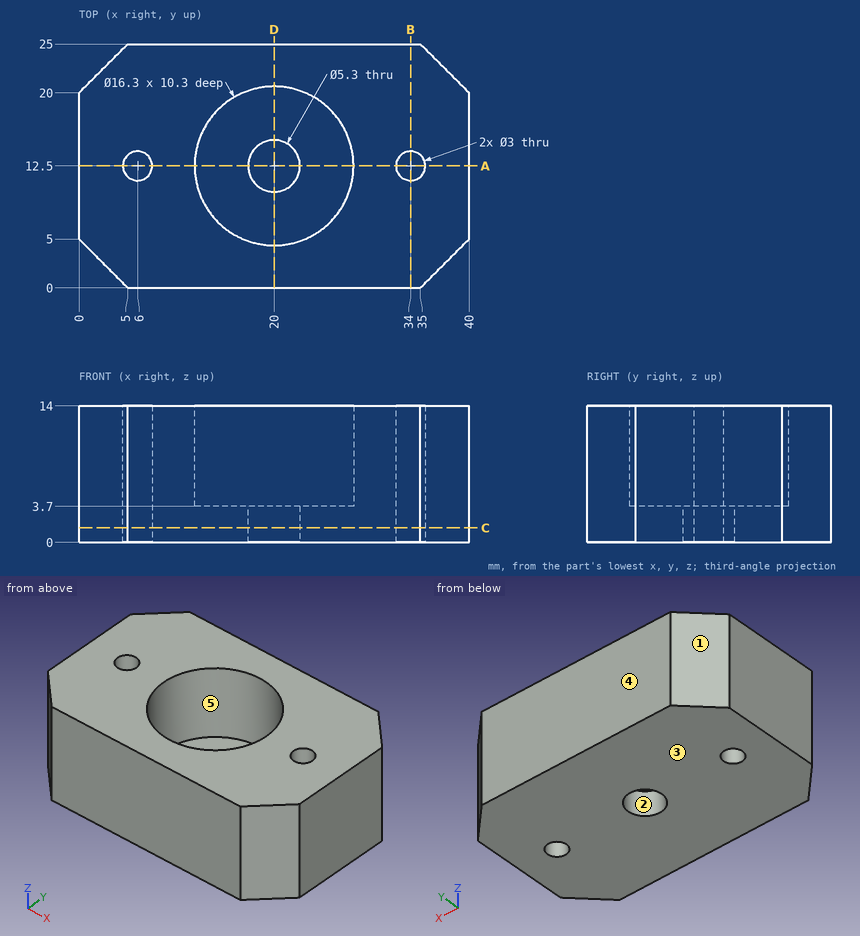
Check sheet for the drawn part. Datum: minimum x, y, z corner. Units: mm. A direction names the side the tool comes from. Coordinates: 2 decimals unless noted, no trailing zeros. Order: outer loops, then holes, each group sorted by start corner. A loop starts at its lowest first (then second) coordinate and runs counter-clockwise, first axis right, second up. Notation, with made-up numbers: M 27,80 L 65,80 A5 ccw 65,87 Z; hole C -34,82.25 d1. An arc over 180 degrees is marked long. One line per question, with ' | ' between items. Start each with the question number.
Item 1: Sectioned sample at B-B on x = 34. Record the cut outline in (y, z).
Item 2: Sectioned sample at C-C on z = 1.5. Record the cut outline in (x, y), and give its area (3 significant figures).
Item 3: Sectioned sample at A-A on y = 12.5. Record the cut outline in (x, z).
Item 4: Sectioned sample at D-D on x = 20. Record the cut outline in (y, z).
Item 5: Access from +Z, -Z, +X, -X, +Y, -Y to the whole of each face (thin tool, end or side, straight path). Record for the marked faces 4 and 5.
Item 6: Gauge pin test, flat ends, axial feed: P1, Ø2.5, axis at x = 6, y = 12.5, coming from the -Z side (3 decimals); P2, Ø7, axis at x = 20, y = 12.5, coming from the +Z side. Record the tip position at first contact, or that the pin passes through.
Item 7: Material ranges on line 1 (Y direction, x = 20, z = 10.25); line 2 (Y direction, x = 6, z = 10.25); line 3 (Z direction, x = 25.5, y = 13.5), recorded low to high.
Item 8: Mould release check, pull along Y, two halves, no side actions. Record for the marked faces 1, 2 and 3: pulls with the +Y half, pulls with the -Y half, needs draft (parallel to the pull), parting line crosses it, or undercut.
Answer below:
1) outline: M 0,0 L 11,0 L 11,14 L 0,14 Z; M 14,0 L 25,0 L 25,14 L 14,14 Z
2) outline: M 0,5 L 5,0 L 35,0 L 40,5 L 40,20 L 35,25 L 5,25 L 0,20 Z; hole C 6,12.5 d3; hole C 20,12.5 d5.3; hole C 34,12.5 d3 | area: 914 mm^2
3) outline: M 0,0 L 4.5,0 L 4.5,14 L 0,14 Z; M 7.5,0 L 17.35,0 L 17.35,3.7 L 11.85,3.7 L 11.85,14 L 7.5,14 Z; M 22.65,0 L 32.5,0 L 32.5,14 L 28.15,14 L 28.15,3.7 L 22.65,3.7 Z; M 35.5,0 L 40,0 L 40,14 L 35.5,14 Z
4) outline: M 0,0 L 9.85,0 L 9.85,3.7 L 4.35,3.7 L 4.35,14 L 0,14 Z; M 15.15,0 L 25,0 L 25,14 L 20.65,14 L 20.65,3.7 L 15.15,3.7 Z
5) face 4: +Z, -Z, +X, -X, +Y | face 5: +Z
6) P1: passes through | P2: stops at z = 3.7
7) line 1: y = 0 to 4.35, 20.65 to 25 | line 2: y = 0 to 11, 14 to 25 | line 3: z = 0 to 3.7
8) face 1: pulls with the +Y half | face 2: undercut | face 3: needs draft
